Autodesk Inventor part; units mm, degrees
ref_plane "YZ Plane" through (0, 0, 0) normal (1, 0, 0) x (0, 1, 0)
ref_plane "XZ Plane" through (0, 0, 0) normal (0, 1, 0) x (-1, 0, 0)
ref_plane "XY Plane" through (0, 0, 0) normal (0, 0, 1) x (1, 0, 0)
sketch "Sketch1" plane through (0, 0, 0) normal (0, 1, 0) x (-1, 0, 0)
  line L0 (0, 0) -> (0, -347.765) construction
  line L1 (-3, 0) -> (-3, -347.765)
  line L2 (3, -347.765) -> (3, 0)
  arc A0 (3, 0) -> (-3, 0) centre (0, 0) ccw
  arc A1 (-3, -347.765) -> (3, -347.765) centre (0, -347.765) ccw
  circle A2 centre (0, 0) radius 1.5
  circle A3 centre (0, -347.765) radius 1.5
  circle A4 centre (0, -131.233) radius 1.5
  circle A5 centre (0, -37.934) radius 1.5
  point P0 (0, -173.8825)
  dimension "d0" = 347.765
  dimension "d1" = 6
  dimension "d2" = 3
  dimension "d3" = 3
  dimension "d6" = 3
  dimension "d7" = 131.233
  dimension "d8" = 3
  dimension "d9" = 37.934
extrude "Extrusion1" add sketch "Sketch1" along normal blind 8
sketch "Sketch2" plane through (0, 8, 0) normal (0, 1, 0) x (1, 0, 0)
  arc A0 (3, 347.765) -> (-3, 347.765) centre (0, 347.765) ccw
  line L0 (-3, 347.765) -> (-3, 0)
  arc A1 (-3, 0) -> (3, 0) centre (0, 0) ccw
  line L1 (3, 0) -> (3, 347.765)
  circle A2 centre (0, 131.233) radius 1.5
  circle A3 centre (0, 37.934) radius 1.5
  circle A4 centre (0, 347.765) radius 1.5
  circle A5 centre (0, 0) radius 1.5
sketch "Sketch3" plane through (0, 8, 0) normal (0, 1, 0) x (1, 0, 0)
  line L0 (-13.5041, 192.6393) -> (33.2898, 192.6393)
  line L1 (33.2898, 192.6393) -> (33.2898, -23.3325)
  line L2 (33.2898, -23.3325) -> (-13.5041, -23.3325)
  line L3 (-13.5041, -23.3325) -> (-13.5041, 192.6393)
  line L4 (-64.7974, 383.8644) -> (82.7834, 383.8644)
  line L5 (82.7834, 383.8644) -> (82.7834, -81.8249)
  line L6 (82.7834, -81.8249) -> (-64.7974, -81.8249)
  line L7 (-64.7974, -81.8249) -> (-64.7974, 383.8644)
  point P0 (0, 0)
extrude "Extrusion2" cut sketch "Sketch3" against normal blind 10
sketch "Sketch4" plane through (0, 8, 0) normal (0, 1, 0) x (1, 0, 0)
  circle A0 centre (0, 0) radius 1.5
  circle A1 centre (0, 37.934) radius 1.5
  circle A2 centre (0, 131.233) radius 1.5
  line L0 (3, 192.6393) -> (-3, 192.6393)
  line L1 (-3, 192.6393) -> (-3, 0)
  arc A3 (-3, 0) -> (3, 0) centre (0, 0) ccw
  line L2 (3, 0) -> (3, 192.6393)
properties part number "Part_10_p2"
Check sheet for the modelled part. Datum: model origin and axes. Units: mm. Round coordinates to 2 decimals unless told otherwise and drop trailing zeros. Order: outer loops, then holes, each group sorted by start corner. A loop starts at its lowest first (then second) coordinate and runs counter-clockwise, first axis right, second up. Notation, with made-up numbers: M -6,-3.75 L 26,-3.75 A26 ccw 26,34.25 Z; hole C 22,-16.75 d1. An arc over 180 degrees is marked long. One line per item, written item: value. Start each with the question number.
1. Release check for a two-part mould opening along Z. For faces 1 (the flat face through (0, 0, -93)), 2 (the cylindrical face through (0.2, 3.94, -39.42)), 3 (the cylindrical face through (0, 4, 3)) record: released by +Z, released by -Z, zero draft, split by the parting line, or undercut.
2. Gauge pin test, flat end, axial feed: P1, Ø3, axis at x = 1, y = 5.5, coming from the +Z side. Record the tip position at first contact, or that the pin passes through.
3. Section check B-B on y = 4. Enter the section's corners in (x, z).
4. Section check A-A on x = 0. Enter the section's corners in (y, z).
5. Scan lines: line 1 along Z through (x, y) = (-0.25, 5); line 2 along Z through (x, y) = (0, 1.5); line 3 along Z through (x, y) = (2.25, 7). Record each from-to range of solid material in increasing order.
Results found:
1. face 1: zero draft
1. face 2: undercut
1. face 3: released by +Z
2. P1: z = 3
3. outline: M -3,-192.64 L 3,-192.64 L 3,0 A3 ccw -3,0 Z; hole C 0,-131.23 d3; hole C 0,-37.93 d3; hole C 0,0 d3
4. outline: M 0,-192.64 L 8,-192.64 L 8,-132.73 L 0,-132.73 Z; M 0,-129.73 L 8,-129.73 L 8,-39.43 L 0,-39.43 Z; M 0,-36.43 L 8,-36.43 L 8,-1.5 L 0,-1.5 Z; M 0,1.5 L 8,1.5 L 8,3 L 0,3 Z
5. line 1: -192.64 to -132.71, -129.75 to -39.41, -36.45 to -1.48, 1.48 to 2.99
5. line 2: -192.64 to -132.73, -129.73 to -39.43, -36.43 to -1.5, 1.5 to 3
5. line 3: -192.64 to 1.98
